from build123d import *

# Parameters (mm, degrees)
F0_R     = 11
F0_R_2   = 4
F1_DEPTH = 3.5
F2_SIZE  = 1
F4_DEPTH = 7.001


# Not quite as in the source:
# - a feature names something its author has since deleted; it is built from what else it names


with BuildPart() as f1:
    # F0 (on Top) → F1 (new body, symmetric)
    with BuildSketch(Plane.XY):
        with BuildLine():
            ThreePointArc((-6, 11.5325625947), (0, 13), (6, 11.5325625947))
            Line((6, 11.5325625947), (6, 25))
            ThreePointArc((6, 25), (0, 19), (-6, 25))
            Line((-6, 25), (-6, 11.5325625947))
        make_face()
        with BuildLine():
            ThreePointArc((-6.9874921777, -10.96243372), (-11.2583302492, -6.5), (-12.9874921777, -0.5701288746))
            Line((-12.9874921777, -0.5701288746), (-24.6506350946, -7.3038475773))
            ThreePointArc((-24.6506350946, -7.3038475773), (-18.6506350946, -7.3038475773), (-15.6506350946, -12.5))
            ThreePointArc((-15.6506350946, -12.5), (-16.4544826719, -15.5), (-18.6506350946, -17.6961524227))
            Line((-18.6506350946, -17.6961524227), (-6.9874921777, -10.96243372))
        make_face()
        with BuildLine():
            Line((24.6506350946, -7.3038475773), (12.9874921777, -0.5701288746))
            ThreePointArc((12.9874921777, -0.5701288746), (11.2583302492, -6.5), (6.9874921777, -10.96243372))
            Line((6.9874921777, -10.96243372), (18.6506350946, -17.6961524227))
            ThreePointArc((18.6506350946, -17.6961524227), (16.4544826719, -9.5), (24.6506350946, -7.3038475773))
        make_face()
        with BuildLine():
            ThreePointArc((12.9874921777, -0.5701288746), (12.9968726683, -0.2851330301), (13, 0))
            ThreePointArc((13, 0), (11.1130553854, 6.7453687816), (6, 11.5325625947))
            ThreePointArc((6, 11.5325625947), (0, 13), (-6, 11.5325625947))
            ThreePointArc((-6, 11.5325625947), (-11.2583302492, 6.5), (-12.9874921777, -0.5701288746))
            ThreePointArc((-12.9874921777, -0.5701288746), (-11.2583302492, -6.5), (-6.9874921777, -10.96243372))
            ThreePointArc((-6.9874921777, -10.96243372), (0, -13), (6.9874921777, -10.96243372))
            ThreePointArc((6.9874921777, -10.96243372), (11.2583302492, -6.5), (12.9874921777, -0.5701288746))
        make_face()
        Circle(F0_R, mode=Mode.SUBTRACT)
        with BuildLine():
            ThreePointArc((-6, 25), (0, 19), (6, 25))
            ThreePointArc((6, 25), (0, 31), (-6, 25))
        make_face()
        with Locations((0, 25)):
            Circle(F0_R_2, mode=Mode.SUBTRACT)
        with BuildLine():
            ThreePointArc((-15.6506350946, -12.5), (-18.6506350946, -7.3038475773), (-24.6506350946, -7.3038475773))
            ThreePointArc((-24.6506350946, -7.3038475773), (-26.8467875173, -15.5), (-18.6506350946, -17.6961524227))
            ThreePointArc((-18.6506350946, -17.6961524227), (-16.4544826719, -15.5), (-15.6506350946, -12.5))
        make_face()
        with Locations((-21.6506350946, -12.5)):
            Circle(F0_R_2, mode=Mode.SUBTRACT)
        with BuildLine():
            ThreePointArc((27.6506350946, -12.5), (26.8467875173, -9.5), (24.6506350946, -7.3038475773))
            ThreePointArc((24.6506350946, -7.3038475773), (16.4544826719, -9.5), (18.6506350946, -17.6961524227))
            ThreePointArc((18.6506350946, -17.6961524227), (24.6506350946, -17.6961524227), (27.6506350946, -12.5))
        make_face()
        with Locations((21.6506350946, -12.5)):
            Circle(F0_R_2, mode=Mode.SUBTRACT)
    extrude(amount=F1_DEPTH, both=True)

    # F2
    f2_edges = [f1.edges().sort_by_distance(p)[0] for p in [
        (-4, 25, 3.5),
        (-11, 0, 3.5),
        (-25.650635, -12.5, 3.5),
        (17.650635, -12.5, 3.5),
        (-25.650635, -12.5, -3.5),
        (-11, 0, -3.5),
        (17.650635, -12.5, -3.5),
        (-4, 25, -3.5),
    ]]
    chamfer(f2_edges, length=F2_SIZE)

    # F3 (on face) → F4 (cut, through all)
    with BuildSketch(Plane.XY.offset(3.5)):
        with BuildLine():
            Line((4, 12.3693168769), (4, 20.527864045))
            ThreePointArc((4, 20.527864045), (0, 19), (-4, 20.527864045))
            Line((-4, 20.527864045), (-4, 12.3693168769))
            ThreePointArc((-4, 12.3693168769), (0, 13), (4, 12.3693168769))
        make_face()
        with BuildLine():
            ThreePointArc((-8.7121426428, -9.6487600536), (-11.2583302492, -6.5), (-12.7121426428, -2.7205568233))
            Line((-12.7121426428, -2.7205568233), (-19.7776517484, -6.7998304074))
            ThreePointArc((-19.7776517484, -6.7998304074), (-16.7907019635, -8.9813283811), (-15.6506350946, -12.5))
            ThreePointArc((-15.6506350946, -12.5), (-15.682473733, -13.117292444), (-15.7776517484, -13.7280336376))
            Line((-15.7776517484, -13.7280336376), (-8.7121426428, -9.6487600536))
        make_face()
        with BuildLine():
            Line((19.7776517484, -6.7998304074), (12.7121426428, -2.7205568233))
            ThreePointArc((12.7121426428, -2.7205568233), (11.2583302492, -6.5), (8.7121426428, -9.6487600536))
            Line((8.7121426428, -9.6487600536), (15.7776517484, -13.7280336376))
            ThreePointArc((15.7776517484, -13.7280336376), (16.4544826719, -9.5), (19.7776517484, -6.7998304074))
        make_face()
    extrude(amount=-F4_DEPTH, mode=Mode.SUBTRACT)


solid = f1.part
The listing builds one solid part. Answer for the finished solid, in the listing's coordinates (mm). A direction names the side the tool comes from. Give positions to 0.01 mm unless a question says otherwise; leave off trailing zeros. Loops run counter-clockwise (first coordinate to the right, second up) from the corner with the lowest first, then second, coordinate; pieces in that order, holes last. Notation, with made-up numbers: (60.5, 55) - (117.5, 55) arc R27 cw to (117.5, 74) - close; hole circle Ø2 at (-13, 16). An arc over 180 degrees is marked (long way). Answer as a JSON object with one key per item and string values.
1. For faces 4 (the flat face through (-6, 18, 0)), 5 (the flat face through (6, 18, 0)), 6 (the flat face through (-16.195, -4.732, 0.049)), determine the directions among +Z, -Z, +X, -X, +Y, -Y from which every point of the face is accessible in a straight line to the end or side of a thin tool.
Determined:
{"face 4": "+Z, -Z, -X, +Y", "face 5": "+Z, -Z, +X, +Y", "face 6": "+Z, -Z"}
2. A cutting plane is placed at D-D (y = -5.5). Give the number of separate pieces and of enclosed holes in the cut face, then the cut area to 3 significant figures.
Determined:
{"separate pieces": "4", "enclosed holes": "0", "area": "85.3 mm²"}
3. Flat-ended cylindrical pins translate along their axes: pin 1 Ø3.5 at (y, z) = (15.5, 0) entering from +X; pin 2 Ø3 at (y, z) = (-2.5, -0.5) entering from -X. Find the tip coordinate at first contact, or state that the pin passes through.
Determined:
{"pin 1": "x = 6", "pin 2": "x = -18.93"}
4. For a pull along X with two mould halves and no side action, classify faces 1 (the cylindrical face through (-11.2, 6.6, 0)), 2 (the flat face through (-2, -12, -3.5)), 3 (the flat face through (-4, 17, 0)) as pulls with the +X half, pulls with the -X half, needs draft (parallel to the pull), parting line crosses it, or undercut.
Determined:
{"face 1": "pulls with the -X half", "face 2": "needs draft", "face 3": "undercut"}
5. A cutting plane is placed at B-B (z = -1.25). Write down the section's boundary in (x, y).
Determined:
{"outline": "(-24.65, -7.3) arc R6 ccw to (-18.65, -17.7) - (-6.99, -10.96) arc R13 ccw to (6.99, -10.96) - (18.65, -17.7) arc R6 ccw to (24.65, -7.3) - (12.99, -0.57) arc R13 ccw to (6, 11.53) - (6, 25) arc R6 ccw to (-6, 25) - (-6, 11.53) arc R13 ccw to (-12.99, -0.57) - close; hole circle Ø8 at (-21.65, -12.5); hole (-19.78, -6.8) arc R6 cw to (-15.78, -13.73) - (-8.71, -9.65) arc R13 cw to (-12.71, -2.72) - close; hole circle Ø22 at (0, 0); hole (-4, 12.37) arc R13 cw to (4, 12.37) - (4, 20.53) arc R6 cw to (-4, 20.53) - close; hole circle Ø8 at (0, 25); hole (8.71, -9.65) - (15.78, -13.73) arc R6 cw to (19.78, -6.8) - (12.71, -2.72) arc R13 cw to start; hole circle Ø8 at (21.65, -12.5)"}
6. A cutting plane is placed at A-A (y = 15). Write down the section's boundary in (x, z), then the cut area to 3 significant figures.
Determined:
{"outline": "(-6, -3.5) - (-4, -3.5) - (-4, 3.5) - (-6, 3.5) - close; (4, -3.5) - (6, -3.5) - (6, 3.5) - (4, 3.5) - close", "area": "28.0 mm²"}
7. A cutting plane is placed at C-C (x = 0). Write down the section's boundary in (y, z).
Determined:
{"outline": "(-13, -3.5) - (-12, -3.5) - (-11, -2.5) - (-11, 2.5) - (-12, 3.5) - (-13, 3.5) - close; (11, -2.5) - (12, -3.5) - (13, -3.5) - (13, 3.5) - (12, 3.5) - (11, 2.5) - close; (19, -3.5) - (20, -3.5) - (21, -2.5) - (21, 2.5) - (20, 3.5) - (19, 3.5) - close; (29, -2.5) - (30, -3.5) - (31, -3.5) - (31, 3.5) - (30, 3.5) - (29, 2.5) - close"}
8. Find the intervals of material crossed by L1, parallel to X at y = -3, z = 0.25; L2, parallel to X at y = -7, z = -2.5; L3, parallel to X at y = 17.5, z = -0.75, in increasing order. Write a range as [from, to].
Determined:
{"L1": "[-17.2, -13.2], [-12.65, -10.58], [10.58, 12.65], [13.2, 17.2]", "L2": "[-24.12, -19.25], [-10.95, -8.49], [8.49, 10.95], [19.25, 24.12]", "L3": "[-6, -4], [4, 6]"}
